```python
from build123d import *

# Parameters (mm, degrees)
SKETCH_1_W          = 30
SKETCH_1_H          = 20
SKETCH_1_W_2        = 28
SKETCH_1_H_2        = 18
EXTRUDE_1_DEPTH     = 75
SKETCH_2_R          = 1.6
CUT_EXTRUDE_1_DEPTH = 80.056941504


with BuildPart() as part:
    # 草图1 → 凸台-拉伸1 (new, symmetric)
    with BuildSketch(Plane.XY):
        Rectangle(SKETCH_1_W, SKETCH_1_H)
        Rectangle(SKETCH_1_W_2, SKETCH_1_H_2, mode=Mode.SUBTRACT)
    extrude(amount=EXTRUDE_1_DEPTH, both=True)

    # 草图2 → 切除-拉伸1 (cut, through all)
    with BuildSketch(Plane(origin=(0, 10, 0), x_dir=(1, 0, 0), z_dir=(0, 1, 0))):
        with Locations(Location((-11, -65, 0), (0, 0, 270))):
            Circle(SKETCH_2_R)
        with Locations(Location((-11, -52.5, 0), (0, 0, 270))):
            Circle(SKETCH_2_R)
        with Locations(Location((-11, -40, 0), (0, 0, 270))):
            Circle(SKETCH_2_R)
        with Locations(Location((-11, -27.5, 0), (0, 0, 270))):
            Circle(SKETCH_2_R)
        with Locations(Location((11, -27.5, 0), (0, 0, 180))):
            Circle(SKETCH_2_R)
        with Locations(Location((11, -40, 0), (0, 0, 180))):
            Circle(SKETCH_2_R)
        with Locations(Location((11, -52.5, 0), (0, 0, 180))):
            Circle(SKETCH_2_R)
        with Locations(Location((11, -65, 0), (0, 0, 180))):
            Circle(SKETCH_2_R)
        with Locations(Location((11, 27.5, 0), (0, 0, 270))):
            Circle(SKETCH_2_R)
        with Locations(Location((-11, 27.5, 0), (0, 0, 180))):
            Circle(SKETCH_2_R)
        with Locations(Location((11, 40, 0), (0, 0, 270))):
            Circle(SKETCH_2_R)
        with Locations(Location((-11, 40, 0), (0, 0, 180))):
            Circle(SKETCH_2_R)
        with Locations(Location((11, 52.5, 0), (0, 0, 270))):
            Circle(SKETCH_2_R)
        with Locations(Location((-11, 52.5, 0), (0, 0, 180))):
            Circle(SKETCH_2_R)
        with Locations(Location((11, 65, 0), (0, 0, 270))):
            Circle(SKETCH_2_R)
        with Locations(Location((-11, 65, 0), (0, 0, 180))):
            Circle(SKETCH_2_R)
        with Locations(Location((-11, -15, 0), (0, 0, 270))):
            Circle(SKETCH_2_R)
        with Locations(Location((11, -15, 0), (0, 0, 180))):
            Circle(SKETCH_2_R)
        with Locations(Location((11, 15, 0), (0, 0, 270))):
            Circle(SKETCH_2_R)
        with Locations(Location((-11, 15, 0), (0, 0, 180))):
            Circle(SKETCH_2_R)
    extrude(amount=-CUT_EXTRUDE_1_DEPTH, mode=Mode.SUBTRACT)


solid = part.part
```
Input: part model. Units: mm. Frame: model coordinates. Give positions to 0.01 mm unless a question says otherwise; leave off trailing zeros. Order: outer loops, then holes, each group sorted by start corner. A loop starts at its lowest first (then second) coordinate and runs counter-clockwise, first axis right, second up. Notation, with made-up numbers: (74, 8.5) - (127, 8.5) arc R30 cw to (127, 43.5) - close; hole circle Ø9 at (-16, 84.5). An arc over 180 degrees is marked (long way). One line per item, written item: value.
1. Draft query along X for faces 1 (the face through (-10.792, -9.493, -63.414)), 2 (the face through (0, -10, 1)). Return one class per face: released by +X, released by -X, zero draft, split by the parting line, or undercut.
Determined:
face 1: undercut
face 2: zero draft
2. Cut plane D-D, the plane x = -2.25. Output: boundary loops of the cut face in (y, z), and give its area (3 significant figures).
Determined:
outline: (-10, -75) - (-9, -75) - (-9, 75) - (-10, 75) - close; (9, -75) - (10, -75) - (10, 75) - (9, 75) - close
area: 300 mm2
3. Pin query (flat end, axial travel): pin 1 Ø2.5 at (x, z) = (-11, -40) entering from -Y. Return the tip coordinate at first contact, or that it passes through.
Determined:
pin 1: through
4. Cut plane C-C, the plane z = -40. Output: boundary loops of the cut face in (x, y), and give its area (3 significant figures).
Determined:
outline: (-15, -10) - (-12.6, -10) - (-12.6, -9) - (-14, -9) - (-14, 9) - (-12.6, 9) - (-12.6, 10) - (-15, 10) - close; (-9.4, -10) - (9.4, -10) - (9.4, -9) - (-9.4, -9) - close; (-9.4, 9) - (9.4, 9) - (9.4, 10) - (-9.4, 10) - close; (12.6, -10) - (15, -10) - (15, 10) - (12.6, 10) - (12.6, 9) - (14, 9) - (14, -9) - (12.6, -9) - close
area: 83.2 mm2
5. Line query: probe 1 along Y at (x, z) = (3.75, 66); probe 2 along X at (y, z) = (9.6, 65); probe 3 along X at (y, z) = (-8.5, -49.5). Output: solid intervals per line, ascending.
Determined:
probe 1: -10 to -9, 9 to 10
probe 2: -15 to -12.6, -9.4 to 9.4, 12.6 to 15
probe 3: -15 to -14, 14 to 15
6. Cut plane B-B, the plane z = -11.5. Output: boundary loops of the cut face in (x, y).
Determined:
outline: (-15, -10) - (15, -10) - (15, 10) - (-15, 10) - close; hole (-14, -9) - (14, -9) - (14, 9) - (-14, 9) - close
7. Cut plane A-A, the plane y = 2.5. Output: boundary loops of the cut face in (x, z).
Determined:
outline: (-15, -75) - (-14, -75) - (-14, 75) - (-15, 75) - close; (14, -75) - (15, -75) - (15, 75) - (14, 75) - close
